Here's how the part is built. I have some questions about the finished solid (model axes, mm). A direction names the side the tool comes from. Coordinates: 2 decimals unless noted, no trailing zeros. Write each loop counter-clockwise with the first axis right and the second up, starting at its lowest first coordinate (ties: lowest second). Pieces come first, ordered by that corner, then holes. Notation, with made-up numbers: (-5, -8) -> (40, -8) arc R23 cw to (40, 22) -> close; hole circle Ø10 at (22.25, 28). An arc over 180 degrees is marked (long way). Put each result on its own line as item: value.
```python
from build123d import *

# Parameters (mm, degrees)
ESQUISSE1_W             = 129.794
ESQUISSE1_H             = 37.9984
BOSS_EXTRU_1_DEPTH      = 2.54
ESQUISSE2_W             = 12.3444
ESQUISSE2_H             = 2.54
BOSS_EXTRU_2_DEPTH      = 129.794
ESQUISSE3_R             = 5.36575
ENL_V_MAT_EXTRU_1_DEPTH = 69.738449364
ESQUISSE4_R             = 1.68275
ENL_V_MAT_EXTRU_2_DEPTH = 77.661883455
ESQUISSE5_R             = 6.35
ENL_V_MAT_EXTRU_3_DEPTH = 2.54
ESQUISSE7_R             = 6
ENL_V_MAT_EXTRU_4_DEPTH = 2.54


with BuildPart() as part:
    # Esquisse1 → Boss.-Extru.1 (new body)
    with BuildSketch(Plane.XY):
        Rectangle(ESQUISSE1_W, ESQUISSE1_H)
    extrude(amount=BOSS_EXTRU_1_DEPTH)

    # Esquisse2 → Boss.-Extru.2 (add)
    with BuildSketch(Plane.ZY.offset(64.897)):
        with Locations((8.7122, 17.7292)):
            Rectangle(ESQUISSE2_W, ESQUISSE2_H)
    extrude(amount=-BOSS_EXTRU_2_DEPTH)

    # Esquisse3 → Enlèv. mat.-Extru.1 (cut, through all)
    with BuildSketch(Plane.XY.offset(2.54)):
        Circle(ESQUISSE3_R)
    extrude(amount=-ENL_V_MAT_EXTRU_1_DEPTH, mode=Mode.SUBTRACT)

    # Esquisse4 → Enlèv. mat.-Extru.2 (cut, through all)
    with BuildSketch(Plane(origin=(0, 18.9992, 0), x_dir=(1, 0, 0), z_dir=(0, 1, 0))):
        with Locations(Location((-38.1, -8.382, 0), (0, 0, 270))):
            Circle(ESQUISSE4_R)
        with Locations(Location((38.1, -8.382, 0), (0, 0, 270))):
            Circle(ESQUISSE4_R)
    extrude(amount=-ENL_V_MAT_EXTRU_2_DEPTH, mode=Mode.SUBTRACT)

    # Esquisse5 → Enlèv. mat.-Extru.3 (cut)
    with BuildSketch(Plane.XY.offset(2.54)):
        with Locations((-39.897, 0)):
            Circle(ESQUISSE5_R)
    extrude(amount=-ENL_V_MAT_EXTRU_3_DEPTH, mode=Mode.SUBTRACT)

    # Esquisse7 → Enlèv. mat.-Extru.4 (cut)
    with BuildSketch(Plane(origin=(0, 0, 0), x_dir=(-1, 0, 0), z_dir=(0, 0, -1))):
        with Locations((-33.02, 0)):
            Circle(ESQUISSE7_R)
    extrude(amount=-ENL_V_MAT_EXTRU_4_DEPTH, mode=Mode.SUBTRACT)


solid = part.part
```
Item 1: For P1, Ø4, axis at x = 28, y = 10, coming from the +Z side; P2, Ø4, axis at x = -38.1, z = 8.382, coming from the -Y side; P3, Ø9.5, axis at x = 0, y = 0, coming from the +Z side, each with a flat end and sliding along its axis, tell me the tip position at first contact or that it passes through.
Output:
P1: stops at z = 2.54
P2: stops at y = 16.46
P3: passes through
Item 2: Imagine slicing it at A-A on x = 0. Write out the boundary of the cut face in (y, z), then the cut area to 3 significant figures.
Output:
outline: (-19, 0) -> (-5.37, 0) -> (-5.37, 2.54) -> (-19, 2.54) -> close; (5.37, 0) -> (19, 0) -> (19, 14.88) -> (16.46, 14.88) -> (16.46, 2.54) -> (5.37, 2.54) -> close
area: 101 mm²
Item 3: Imagine slicing it at D-D on x = 33.02. Write out the boundary of the cut face in (y, z), then the cut area to 3 significant figures.
Output:
outline: (-19, 0) -> (-6, 0) -> (-6, 2.54) -> (-19, 2.54) -> close; (6, 0) -> (19, 0) -> (19, 14.88) -> (16.46, 14.88) -> (16.46, 2.54) -> (6, 2.54) -> close
area: 97.4 mm²
Item 4: Imagine slicing it at B-B on y = 0. Write out the boundary of the cut face in (x, z), then the cut area to 3 significant figures.
Output:
outline: (-64.9, 0) -> (-46.25, 0) -> (-46.25, 2.54) -> (-64.9, 2.54) -> close; (-33.55, 0) -> (-5.37, 0) -> (-5.37, 2.54) -> (-33.55, 2.54) -> close; (5.37, 0) -> (27.02, 0) -> (27.02, 2.54) -> (5.37, 2.54) -> close; (39.02, 0) -> (64.9, 0) -> (64.9, 2.54) -> (39.02, 2.54) -> close
area: 240 mm²
Item 5: Please list where these lines run through material, in increasing order: line 1 along Y through (x, z) = (33.02, 0.55); line 2 along Y through (x, z) = (36.5, 11); line 3 along Z through (x, y) = (-27, 4.5). Write a range as from..to.
Output:
line 1: y = -19..-6, 6..19
line 2: y = 16.46..19
line 3: z = 0..2.54
Item 6: If we mould it in two halves opening along X, with no side actions, what happens to faces 3 (the flat face through (-1, 18.999, 7)), 4 (the flat face through (-64.897, 4, 2)), 5 (the cylindrical face through (39.014, 0.264, 1.252))? For each: released by +X, released by -X, zero draft, split by the parting line, or undercut.
Output:
face 3: zero draft
face 4: released by -X
face 5: undercut
Item 7: Imagine slicing it at C-C on z = 8.75. Write out the boundary of the cut face in (x, y).
Output:
outline: (-64.9, 16.46) -> (-39.74, 16.46) -> (-39.74, 19) -> (-64.9, 19) -> close; (-36.46, 16.46) -> (36.46, 16.46) -> (36.46, 19) -> (-36.46, 19) -> close; (39.74, 16.46) -> (64.9, 16.46) -> (64.9, 19) -> (39.74, 19) -> close
Item 8: Which directions (+Z, -Z, +X, -X, +Y, -Y) give clear straight access to the entire face, cutting with the end or side of a thin tool? Please do faces 1 (the flat face through (64.897, 4, 2)), 2 (the flat face through (-1, 16.459, 9)).
Output:
face 1: +Z, -Z, +X, +Y, -Y
face 2: +Z, +X, -X, -Y
